```python
from build123d import *

# Parameters (mm, degrees)
MODEL_R             = 4
BOSS_EXTRUDE2_DEPTH = 6.35
SKETCH1_W           = 10.16
SKETCH1_H           = 6.35
BOSS_EXTRUDE3_DEPTH = 6.35


with BuildPart() as part:
    # Model → Boss-Extrude2 (new body)
    with BuildSketch(Plane.XY):
        Polygon((419.1, 87.376), (419.1, 71.374), (436.88, 71.374), (436.88, 63.5), (398.78, 0), (0, 0), (0, 95.25), (436.88, 95.25), (436.88, 87.376), align=None)
        with Locations((172.491700482, 88.801347744)):
            Circle(MODEL_R, mode=Mode.SUBTRACT)
        with Locations((330.479700482, 66.449347744)):
            Circle(MODEL_R, mode=Mode.SUBTRACT)
        with BuildLine():
            Line((312.685453403, 15.123873353), (345.228141797, 48.298807013))
            ThreePointArc((345.228141797, 48.298807013), (345.756846653, 51.060789203), (343.414895332, 52.617496771))
            Line((343.414895332, 52.617496771), (310.872206937, 52.617496771))
            ThreePointArc((310.872206937, 52.617496771), (309.076155713, 51.873547995), (308.332206937, 50.077496771))
            Line((308.332206937, 50.077496771), (308.332206937, 16.902563111))
            ThreePointArc((308.332206937, 16.902563111), (309.911490023, 14.551260704), (312.685453403, 15.123873353))
        make_face(mode=Mode.SUBTRACT)
        with BuildLine():
            Line((171.232102448, 6.35), (215.9, 6.35))
            ThreePointArc((215.9, 6.35), (220.390128061, 8.209871939), (222.25, 12.7))
            Line((222.25, 12.7), (222.25, 57.367897552))
            ThreePointArc((222.25, 57.367897552), (220.682015918, 59.714551565), (217.913948776, 59.163948776))
            Line((217.913948776, 59.163948776), (169.436051224, 10.686051224))
            ThreePointArc((169.436051224, 10.686051224), (168.885448435, 7.917984082), (171.232102448, 6.35))
        make_face(mode=Mode.SUBTRACT)
        with BuildLine():
            Line((234.95, 57.367897552), (234.95, 12.7))
            ThreePointArc((234.95, 12.7), (236.809871939, 8.209871939), (241.3, 6.35))
            Line((241.3, 6.35), (285.967897552, 6.35))
            ThreePointArc((285.967897552, 6.35), (288.314551565, 7.917984082), (287.763948776, 10.686051224))
            Line((287.763948776, 10.686051224), (239.286051224, 59.163948776))
            ThreePointArc((239.286051224, 59.163948776), (236.517984082, 59.714551565), (234.95, 57.367897552))
        make_face(mode=Mode.SUBTRACT)
        with BuildLine():
            Line((294.113948776, 17.036051224), (245.636051224, 65.513948776))
            ThreePointArc((245.636051224, 65.513948776), (245.085448435, 68.282015918), (247.432102448, 69.85))
            Line((247.432102448, 69.85), (292.1, 69.85))
            ThreePointArc((292.1, 69.85), (296.590128061, 67.990128061), (298.45, 63.5))
            Line((298.45, 63.5), (298.45, 18.832102448))
            ThreePointArc((298.45, 18.832102448), (296.882015918, 16.485448435), (294.113948776, 17.036051224))
        make_face(mode=Mode.SUBTRACT)
        with BuildLine():
            Line((323.632102448, 6.35), (368.3, 6.35))
            ThreePointArc((368.3, 6.35), (372.790128061, 8.209871939), (374.65, 12.7))
            Line((374.65, 12.7), (374.65, 57.367897552))
            ThreePointArc((374.65, 57.367897552), (373.082015918, 59.714551565), (370.313948776, 59.163948776))
            Line((370.313948776, 59.163948776), (321.836051224, 10.686051224))
            ThreePointArc((321.836051224, 10.686051224), (321.285448435, 7.917984082), (323.632102448, 6.35))
        make_face(mode=Mode.SUBTRACT)
        with BuildLine():
            Line((18.832102448, 6.35), (63.5, 6.35))
            ThreePointArc((63.5, 6.35), (67.990128061, 8.209871939), (69.85, 12.7))
            Line((69.85, 12.7), (69.85, 57.367897552))
            ThreePointArc((69.85, 57.367897552), (68.282015918, 59.714551565), (65.513948776, 59.163948776))
            Line((65.513948776, 59.163948776), (17.036051224, 10.686051224))
            ThreePointArc((17.036051224, 10.686051224), (16.485448435, 7.917984082), (18.832102448, 6.35))
        make_face(mode=Mode.SUBTRACT)
        with BuildLine():
            Line((82.55, 57.367897552), (82.55, 12.7))
            ThreePointArc((82.55, 12.7), (84.409871939, 8.209871939), (88.9, 6.35))
            Line((88.9, 6.35), (133.567897552, 6.35))
            ThreePointArc((133.567897552, 6.35), (135.914551565, 7.917984082), (135.363948776, 10.686051224))
            Line((135.363948776, 10.686051224), (86.886051224, 59.163948776))
            ThreePointArc((86.886051224, 59.163948776), (84.117984082, 59.714551565), (82.55, 57.367897552))
        make_face(mode=Mode.SUBTRACT)
        with BuildLine():
            Line((93.236051224, 65.513948776), (141.713948776, 17.036051224))
            ThreePointArc((141.713948776, 17.036051224), (144.482015918, 16.485448435), (146.05, 18.832102448))
            Line((146.05, 18.832102448), (146.05, 63.5))
            ThreePointArc((146.05, 63.5), (144.190128061, 67.990128061), (139.7, 69.85))
            Line((139.7, 69.85), (95.032102448, 69.85))
            ThreePointArc((95.032102448, 69.85), (92.685448435, 68.282015918), (93.236051224, 65.513948776))
        make_face(mode=Mode.SUBTRACT)
        with BuildLine():
            Line((163.086051224, 17.036051224), (211.563948776, 65.513948776))
            ThreePointArc((211.563948776, 65.513948776), (212.114551565, 68.282015918), (209.767897552, 69.85))
            Line((209.767897552, 69.85), (165.1, 69.85))
            ThreePointArc((165.1, 69.85), (160.609871939, 67.990128061), (158.75, 63.5))
            Line((158.75, 63.5), (158.75, 18.832102448))
            ThreePointArc((158.75, 18.832102448), (160.317984082, 16.485448435), (163.086051224, 17.036051224))
        make_face(mode=Mode.SUBTRACT)
        with BuildLine():
            Line((6.35, 63.5), (6.35, 18.832102448))
            ThreePointArc((6.35, 18.832102448), (7.917984082, 16.485448435), (10.686051224, 17.036051224))
            Line((10.686051224, 17.036051224), (59.163948776, 65.513948776))
            ThreePointArc((59.163948776, 65.513948776), (59.714551565, 68.282015918), (57.367897552, 69.85))
            Line((57.367897552, 69.85), (12.7, 69.85))
            ThreePointArc((12.7, 69.85), (8.209871939, 67.990128061), (6.35, 63.5))
        make_face(mode=Mode.SUBTRACT)
    extrude(amount=BOSS_EXTRUDE2_DEPTH)

    # Sketch1 → Boss-Extrude3 (add)
    with BuildSketch(Plane.XY.offset(6.35)):
        with Locations((74.93, -3.175)):
            Rectangle(SKETCH1_W, SKETCH1_H)
        with Locations((227.33, -3.175)):
            Rectangle(SKETCH1_W, SKETCH1_H)
    extrude(amount=-BOSS_EXTRUDE3_DEPTH)


solid = part.part
```
Here's how the part is built. I have some questions about the finished solid (model axes, mm). A direction names the side the tool comes from. Coordinates: 2 decimals unless noted, no trailing zeros. Loops run counter-clockwise (first coordinate to the right, second up) from the corner with the lowest first, then second, coordinate; pieces in that order, holes last. Notation, with made-up numbers: (57, 68) - (71, 68) arc R29 ccw to (71, 98) - close; hole circle Ø6 at (51.5, 81). An arc over 180 degrees is marked (long way). Return JSON: item names as keys, results as strings. Group by question number.
Item 1: If we section it at A-A on x = 351: Write out the boundary of the cut face in (y, z).
Item 2: If we section it at B-B on x = 275: Write out the boundary of the cut face in (y, z).
Item 3: Will these pins go through, and if not, where does the flat tip stop? P1, Ø2, axis at x = 93, z = 2.5, coming from the -Y side; P2, Ø1.9, axis at x = 425.5, z = 3.5, coming from the -Y side; P3, Ø3, axis at y = 36, z = 3, coming from the +X side.
Item 4: I need wall thicknesses on line 1 (X direction, y = 67.5, z = 1.25); line 2 (Y direction, x = 345, z = 3.25); line 3 (X direction, y = 10, z = 1.5). Which ranges of each line are inside material? Lowest first, please. Write a range as from..to.
Item 5: If we section it at C-C on y = 33: State how many separate pieces and enclosed holes the cut face has, and give its area (3 significant figures).
Item 6: We'd pull the mould along Y, two halves only. Please class faces 1 (the face through (418.1, 32.2, 3.1)), 2 (the face through (194.01, 35.26, 3.13)), 3 (the face through (221, 68, 0)): +Y half, -Y half, draft (parallel to the pull), parting line (faces both ways), or undercut.
Item 7: On a 3-axis mill with a long thin cutter (end or side, diameter ignored), from which of +Z, -Z, +X, -X, +Y, -Y can I reach the whole of each face in a straight line? I mean faces 4 (the face through (221, 68, 6.35)), 5 (the face through (41.61, 35.26, 3.13)). Say none if no direction works.
Calculated:
{
 "1": {"outline": "(0, 0) - (6.35, 0) - (6.35, 6.35) - (0, 6.35) - close; (39.85, 0) - (95.25, 0) - (95.25, 6.35) - (39.85, 6.35) - close"},
 "2": {"outline": "(0, 0) - (6.35, 0) - (6.35, 6.35) - (0, 6.35) - close; (23.45, 0) - (36.15, 0) - (36.15, 6.35) - (23.45, 6.35) - close; (69.85, 0) - (95.25, 0) - (95.25, 6.35) - (69.85, 6.35) - close"},
 "3": {"P1": "stops at y = 0", "P2": "stops at y = 42.95", "P3": "stops at x = 421.28"},
 "4": {"line 1": "x = 0..7.77, 59.9..92.5, 144.63..160.17, 212.3..244.9, 297.03..326.62, 334.34..436.88", "line 2": "y = 0..6.35, 33.85..48.07, 52.06..95.25", "line 3": "x = 0..16.55, 69.25..83.15, 135.85..168.95, 221.65..235.55, 288.25..321.35, 374.05..404.78"},
 "5": {"separate pieces": "11", "enclosed holes": "0", "area": "1,030 mm^2"},
 "6": {"face 1": "-Y half", "face 2": "undercut", "face 3": "draft"},
 "7": {"face 4": "+Z, +X, -X, +Y, -Y", "face 5": "+Z, -Z"}
}
